Design review of the part built by this model. Coordinates are the model's own, in mm. Give positions to 0.01 mm unless a question says otherwise; leave off trailing zeros. Loops run counter-clockwise (first coordinate to the right, second up) from the corner with the lowest first, then second, coordinate; pieces in that order, holes last. Notation, with made-up numbers: (79, -20.5) -> (100, -20.5) arc R23 ccw to (100, 1.5) -> close; hole circle Ø1 at (89, 72). An arc over 180 degrees is marked (long way). Answer in a Markdown table with one row per item. Add a question column.
(1) Consider section A-A on x = 0.85. Write out the cut boundary in (y, z).
(2) Consider section B-B on z = 128.5. Write out the cut boundary in (x, y).
(3) For pin 1 (6 mm diameter, centred on y = 3, z = -135, fed in from -X); pin 2 (1 mm diameter, centred on x = 1.5, y = -3.5, fed in from -Z); pin 3 (0.9 mm diameter, centred on x = 1, z = -48, fed in from +Y); pin 4 (0.9 mm diameter, centred on x = 1.5, z = 27, fed in from -Y), all flat-tipped, find the tip position at first contact; note any pin that passes through.
(4) Draft analysis for pull direction Z (two halves, no side actions). For faces 1 (the flat face through (3, 0, -2)), 2 (the cylindrical face through (1, 0, -171)), state which applies: +Z half, -Z half, draft (parallel to the pull), parting line (faces both ways), or undercut.
(5) For line 1 (Y direction, x = 2.05, z = 165); line 2 (Y direction, x = 0.1, z = -7); line 3 (Z direction, x = 1.3, y = 4.75), list the stretches that pass through material, from the lowest coordinate up.
from build123d import *

# Parameters (mm, degrees)
SKETCH1_R           = 6
SKETCH1_R_2         = 1.5
SKETCH1_W           = 160.527864045
SKETCH1_H           = 8
BOSS_EXTRUDE1_DEPTH = 3
FILLET1_R           = 10
FILLET2_R           = 10
FILLET3_R           = 10
FILLET4_R           = 10


with BuildPart() as part:
    # Sketch1 → Boss-Extrude1 (new body)
    # profile 1 of 2: a face of its own
    with BuildSketch(Plane(origin=(0, 0, 0), x_dir=(0, 0, -1), z_dir=(1, 0, 0))):
        with Locations((165, 0)):
            Circle(SKETCH1_R)
        with Locations((165, 0)):
            Circle(SKETCH1_R_2, mode=Mode.SUBTRACT)
    # profile 2 of 2: a face of its own
    with BuildSketch(Plane(origin=(0, 0, 0), x_dir=(0, 0, -1), z_dir=(1, 0, 0))):
        with Locations((80.263932023, 0)):
            Rectangle(SKETCH1_W, SKETCH1_H)
    boss_extrude1 = extrude(amount=BOSS_EXTRUDE1_DEPTH)

    # Mirror1: Boss-Extrude1 across plane
    add(boss_extrude1.mirror(Plane.XY))

    # Fillet1
    fillet1_edges = [part.edges().sort_by_distance(p)[0] for p in [
        (1.5, 4, 160.527864045),
    ]]
    fillet(fillet1_edges, radius=FILLET1_R)

    # Fillet2
    fillet2_edges = [part.edges().sort_by_distance(p)[0] for p in [
        (1.5, -4, 160.527864045),
    ]]
    fillet(fillet2_edges, radius=FILLET2_R)

    # Fillet3
    fillet3_edges = [part.edges().sort_by_distance(p)[0] for p in [
        (1.5, -4, -160.527864045),
    ]]
    fillet(fillet3_edges, radius=FILLET3_R)

    # Fillet4
    fillet4_edges = [part.edges().sort_by_distance(p)[0] for p in [
        (1.5, 4, -160.527864045),
    ]]
    fillet(fillet4_edges, radius=FILLET4_R)


solid = part.part
Values follow:
| question | item | result |
|---|---|---|
| 1 | outline | (-5.25, -162.1) arc R6 ccw (long way) to (5.25, -162.1) arc R10 cw to (4, -157.25) -> (4, 157.25) arc R10 cw to (5.25, 162.1) arc R6 ccw (long way) to (-5.25, 162.1) arc R10 cw to (-4, 157.25) -> (-4, -157.25) arc R10 cw to start; hole circle Ø3 at (0, -165); hole circle Ø3 at (0, 165) |
| 2 | outline | (0, -4) -> (3, -4) -> (3, 4) -> (0, 4) -> close |
| 3 | pin 1 | x = 0 |
| 3 | pin 2 | z = -170.2 |
| 3 | pin 3 | y = 4 |
| 3 | pin 4 | y = -4 |
| 4 | face 1 | draft |
| 4 | face 2 | undercut |
| 5 | line 1 | -6 to -1.5, 1.5 to 6 |
| 5 | line 2 | -4 to 4 |
| 5 | line 3 | -168.67 to -161.05, 161.05 to 168.67 |
